```python
from build123d import *

# Parameters (mm, degrees)
BOSS_EXTRU_1_DEPTH         = 9
CONG_1_R                   = 6
CONG_2_R                   = 4
BOSS_EXTRU_2_DEPTH         = 18
R_P_TITION_LIN_AIRE1_COUNT = 6
R_P_TITION_LIN_AIRE1_PITCH = 6
ENL_V_MAT_EXTRU_1_DEPTH    = 131.397228353
ENL_V_MAT_EXTRU_2_DEPTH    = 10
ESQUISSE5_R                = 1.5
ENL_V_MAT_EXTRU_3_DEPTH    = 131.397228353
ESQUISSE7_R                = 1.75
BOSS_EXTRU_3_DEPTH         = 3
ESQUISSE8_R                = 1.25
ENL_V_MAT_EXTRU_4_DEPTH    = 1
ESQUISSE9_R                = 1.25
ENL_V_MAT_EXTRU_5_DEPTH    = 1
ENL_V_MAT_EXTRU_6_DEPTH    = 1


with BuildPart() as part:
    # Esquisse1 → Boss.-Extru.1 (new, symmetric)
    with BuildSketch(Plane(origin=(0, 0, 0), x_dir=(1, 0, 0), z_dir=(0, 1, 0))):
        with BuildLine():
            ThreePointArc((3.322818072, -58.807369293), (12.01141452, -57.437534528), (12.729634722, -66.204079757))
            Line((12.729634722, -66.204079757), (5.979619104, -73.58224275))
            Line((5.979619104, -73.58224275), (5.979619104, -123.58224275))
            Line((5.979619104, -123.58224275), (-5.020380896, -123.58224275))
            Line((-5.020380896, -123.58224275), (-5.020380896, -116.58224275))
            Line((-5.020380896, -116.58224275), (-12.254374663, -87.467481302))
            Line((-12.254374663, -87.467481302), (-24.674189245, -83.627142028))
            Line((-24.674189245, -83.627142028), (-21.720082111, -74.073438503))
            Line((-21.720082111, -74.073438503), (-7.162701387, -70.45644162))
            Line((-7.162701387, -70.45644162), (0.090794599, -70.45644162))
            Line((0.090794599, -70.45644162), (3.322818072, -58.807369293))
        make_face()
        Polygon((-7.162701387, -70.45644162), (-15.931386255, 0), (-39.070246498, -6.371275122), (-18.378388293, -73.243145172), align=None)
    extrude(amount=BOSS_EXTRU_1_DEPTH, both=True)

    # Congé1
    cong_1_edges = [part.edges().sort_by_distance(p)[0] for p in [
        (-39.070246498, 0, 6.371275122),
        (-15.931386255, 0, 0),
    ]]
    fillet(cong_1_edges, radius=CONG_1_R)

    # Congé2
    cong_2_edges = [part.edges().sort_by_distance(p)[0] for p in [
        (-5.020380896, 0, 123.58224275),
        (-24.674189245, 0, 83.627142028),
        (-21.720082111, 0, 74.073438503),
    ]]
    fillet(cong_2_edges, radius=CONG_2_R)

    # Esquisse2 → Boss.-Extru.2 (add, through all)
    with BuildSketch(Plane(origin=(0, 9, 0), x_dir=(1, 0, 0), z_dir=(0, 1, 0))):
        Polygon((5.979619104, -116.58224275), (5.979619104, -118.58224275), (9.979619104, -118.58224275), align=None)
        Polygon((5.979619104, -118.58224275), (5.979619104, -120.58224275), (9.979619104, -118.58224275), align=None)
    boss_extru_2 = extrude(amount=-BOSS_EXTRU_2_DEPTH)

    # Répétition linéaire1: Boss.-Extru.2 ×6
    with Locations(*[(0, 0, -i * R_P_TITION_LIN_AIRE1_PITCH) for i in range(1, R_P_TITION_LIN_AIRE1_COUNT)]):
        add(boss_extru_2)

    # Esquisse3 → Enlèv. mat.-Extru.1 (cut, through all)
    with BuildSketch(Plane(origin=(0, 9, 0), x_dir=(1, 0, 0), z_dir=(0, 1, 0))):
        Polygon((4.500460605, -114.682587681), (4.500460605, -89.682587681), (-10.499539395, -89.682587681), align=None)
    extrude(amount=-ENL_V_MAT_EXTRU_1_DEPTH, mode=Mode.SUBTRACT)

    # Esquisse4 → Enlèv. mat.-Extru.2 (cut)
    with BuildSketch(Plane(origin=(-32.010787668, 0, 7.953554381), x_dir=(0.24113312555809657, 0, 0.9704920482716916), z_dir=(-0.9704920482716917, 0, 0.2411331255580966))):
        Polygon((87.931559422, 6), (87.931559422, -6), (105.931559422, -3.5), (105.931559422, 3.5), align=None)
    extrude(amount=-ENL_V_MAT_EXTRU_2_DEPTH, mode=Mode.SUBTRACT)

    # Esquisse5 → Enlèv. mat.-Extru.3 (cut, through all)
    with BuildSketch(Plane(origin=(0, 9, 0), x_dir=(1, 0, 0), z_dir=(0, 1, 0))):
        with Locations(Location((-31.508218287, -10.512370957, 0), (0, 0, 270))):
            Circle(ESQUISSE5_R)
    extrude(amount=-ENL_V_MAT_EXTRU_3_DEPTH, mode=Mode.SUBTRACT)

    # Esquisse7 → Boss.-Extru.3 (add)
    with BuildSketch(Plane(origin=(0, 9, 0), x_dir=(1, 0, 0), z_dir=(0, 1, 0))):
        with Locations(Location((-19.671064982, -80.987303471, 0), (0, 0, 270))):
            Circle(ESQUISSE7_R)
        with Locations(Location((8.302736926, -62.154070386, 0), (0, 0, 270))):
            Circle(ESQUISSE7_R)
    boss_extru_3 = extrude(amount=BOSS_EXTRU_3_DEPTH)

    # Esquisse8 → Enlèv. mat.-Extru.4 (cut)
    with BuildSketch(Plane(origin=(0, 12, 0), x_dir=(1, 0, 0), z_dir=(0, 1, 0))):
        with Locations(Location((-19.671064982, -80.987303471, 0), (0, 0, 270))):
            Circle(ESQUISSE8_R)
    enl_v_mat_extru_4 = extrude(amount=-ENL_V_MAT_EXTRU_4_DEPTH, mode=Mode.SUBTRACT)

    # Esquisse9 → Enlèv. mat.-Extru.5 (cut)
    with BuildSketch(Plane(origin=(0, 12, 0), x_dir=(1, 0, 0), z_dir=(0, 1, 0))):
        with Locations(Location((8.302736926, -62.154070386, 0), (0, 0, 270))):
            Circle(ESQUISSE9_R)
    enl_v_mat_extru_5 = extrude(amount=-ENL_V_MAT_EXTRU_5_DEPTH, mode=Mode.SUBTRACT)

    # Esquisse10 → Enlèv. mat.-Extru.6 (cut)
    with BuildSketch(Plane(origin=(0, 9, 0), x_dir=(1, 0, 0), z_dir=(0, 1, 0))):
        with BuildLine():
            Line((-28.470192989, -18.951500143), (-15.418940428, -61.130489417))
            ThreePointArc((-15.418940428, -61.130489417), (-16.281236664, -62.765523067), (-17.916270315, -61.903226831))
            Line((-17.916270315, -61.903226831), (-30.967522877, -19.724237556))
            ThreePointArc((-30.967522877, -19.724237556), (-30.10522664, -18.089203906), (-28.470192989, -18.951500143))
        make_face()
    enl_v_mat_extru_6 = extrude(amount=-ENL_V_MAT_EXTRU_6_DEPTH, mode=Mode.SUBTRACT)

    # Symétrie1: Boss.-Extru.3, Enlèv. mat.-Extru.4, Enlèv. mat.-Extru.5, Enlèv. mat.-Extru.6 across plane
    add(boss_extru_3.mirror(Plane.ZX))
    add(enl_v_mat_extru_4.mirror(Plane.ZX), mode=Mode.SUBTRACT)
    add(enl_v_mat_extru_5.mirror(Plane.ZX), mode=Mode.SUBTRACT)
    add(enl_v_mat_extru_6.mirror(Plane.ZX), mode=Mode.SUBTRACT)


solid = part.part
```
Could you check a few things on this model? Use its own coordinates, in mm. A direction names the side the tool comes from. Give positions to 0.01 mm unless a question says otherwise; leave off trailing zeros. Loops run counter-clockwise (first coordinate to the right, second up) from the corner with the lowest first, then second, coordinate; pieces in that order, holes last. Notation, with made-up numbers: (50, 29) - (87, 29) arc R16 ccw to (87, 53) - close; hole circle Ø11 at (23, 59.25). An arc over 180 degrees is marked (long way). Answer in a Markdown table with one row per item. Add a question column.
Q1. For pin 1 (6 mm diameter, centred on x = -15.5, y = -5.5, fed in from +Z); pin 2 (6 mm diameter, centred on y = -9.5, z = 50.5, fed in from -X); pin 3 (9 mm diameter, centred on y = 4, z = 98.5, fed in from -X), each with a flat end and sliding along its axis, tell me the tip position at first contact or that it passes through.
Q2. We'd pull the mould along X, two halves only. Please class faces 5 (the face through (8.008, 0.126, 93.596)), 6 (the face through (8, 11, 62)), 7 (the face through (8.358, -11.507, 60.905)), 8 (the face through (-11, -9, 58)): +X half, -X half, draft (parallel to the pull), parting line (faces both ways), or undercut.
Q3. Please list where these lines run through material, in increasing order: L1, parallel to Y at x = -11.5, z = 57; L2, parallel to X at y = 4, z = 59; L3, parallel to X at y = -8.25, z = 90.5. Write a range as from..to.
Q4. If we section it at A-A (z = 21.5): List the corners of the cut face in (x, y) for me, plus the area to 3 significant figures.
Q5. Which directions (+Z, -Z, +X, -X, +Y, -Y) give clear straight access to the entire face, cutting with the end or side of a thin tool? Please do faces 1 (the face through (7.63, 10.48, 63.77)), 2 (the face through (-18.488, -10.479, 79.697)), 3 (the face through (-27.94, 0.13, 42.34)), 4 (the face through (7.952, 0.126, 89.596)).
The answers:
| question | item | result |
|---|---|---|
| 1 | pin 1 | stops at z = 87.39 |
| 1 | pin 2 | stops at x = -26.33 |
| 1 | pin 3 | stops at x = -10.53 |
| 2 | face 5 | +X half |
| 2 | face 6 | undercut |
| 2 | face 7 | undercut |
| 2 | face 8 | draft |
| 3 | L1 | y = -9..9 |
| 3 | L2 | x = -22.79..-8.59, 3.27..13.41 |
| 3 | L3 | x = -11.5..-10.01, 4.5..6.14 |
| 4 | outline | (-34.39, -9) - (-30.42, -9) - (-30.42, -8) - (-27.68, -8) - (-27.68, -9) - (-13.26, -9) - (-13.26, 9) - (-27.68, 9) - (-27.68, 8) - (-30.42, 8) - (-30.42, 9) - (-34.39, 9) - close |
| 4 | area | 375 mm^2 |
| 5 | face 1 | +Y |
| 5 | face 2 | -Y |
| 5 | face 3 | -X, +Y, -Y |
| 5 | face 4 | +X, +Y, -Y |
